```python
from build123d import *

# Parameters (mm, degrees)
ESQUISSE2_R   = 12.5
ESQUISSE2_R_2 = 11.5


with BuildPart() as part:
    # Balayage1: sweep along a curve in space
    with BuildLine() as balayage1_path:
        Line((-46.602540378, 0, 0), (0, 0, 0))
        ThreePointArc((-46.602540378, 0, 0), (-59.543492634, 1.703708686, 0), (-71.602540378, 6.698729811, 0))
        Line((-71.602540378, 6.698729811, 0), (-106.126093697, 26.630912613, 0))
        ThreePointArc((-106.126093697, 26.630912613, 0), (-120.302247758, 32.589576105, -1.403267638), (-135.054070374, 34.641016151, -5.479233521))
        Line((-135.054070374, 34.641016151, -5.479233521), (-299.933342618, 34.641016151, -65.490380865))
    # Esquisse2 → Balayage1 (sweep)
    with BuildSketch(Plane(origin=(0, 0, 0), x_dir=(0, 0, -1), z_dir=(1, 0, 0))):
        Circle(ESQUISSE2_R)
        Circle(ESQUISSE2_R_2, mode=Mode.SUBTRACT)
    balayage1 = sweep(path=balayage1_path.line)

    # Symétrie1: Balayage1 across plane
    add(balayage1.mirror(Plane(origin=(0, 0, 0), x_dir=(0, 0, 1), z_dir=(1, 0, 0))))


solid = part.part
```
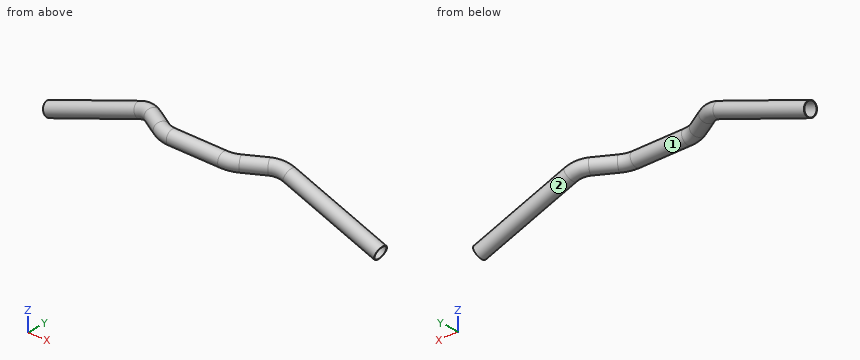
Design review of the part built by this model. Coordinates are the model's own, in mm. Face numbers are marked on the shaded views. Coordinates: 2 decimals unless noted, no trailing zeros. Order: outer loops, then holes, each group sorted by start corner. A loop starts at its lowest first (then second) coordinate and runs counter-clockwise, first axis right, second up. Notation, with made-up numbers: M -27,7.25 L -21,7.25 A36 ccw -21,46.25 Z; hole C -1.5,52.25 d5. An arc over 180 degrees is marked long. Answer as a JSON object with one key per item and string values. Group by question number.
1) Add section A-A, the plane x = 20. Write out the cut boundary in (y, z).
2) Mouldability with a two-part tool opening along X and no side actions: class the marked faces 1 and 2 as pulls with the +X half, pulls with the -X half, needs draft (parallel to the pull), parting line crosses it, or undercut.
3) For pin 1 (5 mm diameter, centred on x = -228, z = -27, fed in from +Y); pin 2 (10 mm diameter, centred on x = 89.5, y = 29.5, fed in from +Z); pin 3 (12 mm diameter, centred on y = 26.5, z = -67, fed in from +X); pin 4 (1 mm diameter, centred on x = 4.5, y = 14.5, fed in from +Z), all flat-tipped, find the tip position at first contact; note any pin that passes through.
4) Wall thickness on L1, parallel to Y at x = -17, z = 0; L2, parallel to Y at x = 253, z = -55; L3, parallel to Z at x = -63, y = 9.5: over which ranges is each line inside the solid? List them lowest first.
Computed values:
{
 "1": {"outline": "C 0,0 d25; hole C 0,0 d23"},
 "2": {"face 1": "undercut", "face 2": "undercut"},
 "3": {"pin 1": "stops at y = 43.25", "pin 2": "stops at z = 11.07", "pin 3": "stops at x = 301.36", "pin 4": "passes through"},
 "4": {"L1": "y = -12.5 to -11.5, 11.5 to 12.5", "L2": "y = 23.78 to 24.95, 44.33 to 45.5", "L3": "z = -10.79 to -9.62, 9.62 to 10.79"}
}
